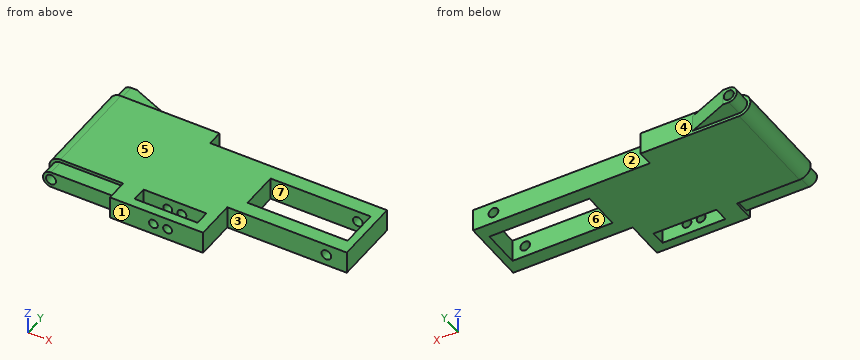
```python
from build123d import *

# Parameters (mm, degrees)
SKETCH_W        = 91.1
SKETCH_H        = 44.5
PAD_DEPTH       = 3.55
POCKET_DEPTH    = 7.101
SKETCH002_W     = 38
SKETCH002_H     = 12.8
POCKET001_DEPTH = 7.101
SKETCH003_W     = 23.5
SKETCH003_H     = 2
POCKET002_DEPTH = 7.101
SKETCH004_W     = 31.8
SKETCH004_H     = 12.2
POCKET003_DEPTH = 7.101
SKETCH005_W     = 20
SKETCH005_H     = 4.7
POCKET004_DEPTH = 7.101
POCKET005_DEPTH = 42.501
POCKET006_DEPTH = 5
POCKET007_DEPTH = 5.5
SKETCH009_R     = 1.6
POCKET008_DEPTH = 42.501
SKETCH010_R     = 1.55
POCKET009_DEPTH = 44.501
SKETCH011_R     = 1.4
POCKET010_DEPTH = 16


with BuildPart() as part:
    # Sketch → Pad (new body, symmetric)
    with BuildSketch(Plane.XY):
        with Locations((45.55, 0)):
            Rectangle(SKETCH_W, SKETCH_H)
    extrude(amount=PAD_DEPTH, both=True)

    # Sketch001 → Pocket (cut, through all)
    with BuildSketch(Plane.XY.offset(3.55)):
        Polygon((5.4, 22.25), (91.1, 22.25), (91.1, 11.85), (34.9, 11.85), (34.9, 16.75), (18.4, 16.75), align=None)
    extrude(amount=-POCKET_DEPTH, mode=Mode.SUBTRACT)

    # Sketch002 → Pocket001 (cut, through all)
    with BuildSketch(Plane.XY.offset(3.55)):
        with Locations((72.1, -15.85)):
            Rectangle(SKETCH002_W, SKETCH002_H)
    extrude(amount=-POCKET001_DEPTH, mode=Mode.SUBTRACT)

    # Sketch003 → Pocket002 (cut, through all)
    with BuildSketch(Plane.XY.offset(3.55)):
        with Locations((11.75, -21.25)):
            Rectangle(SKETCH003_W, SKETCH003_H)
    extrude(amount=-POCKET002_DEPTH, mode=Mode.SUBTRACT)

    # Sketch004 → Pocket003 (cut, through all)
    with BuildSketch(Plane.XY.offset(3.55)):
        with Locations((72.75, 1.15)):
            Rectangle(SKETCH004_W, SKETCH004_H)
    extrude(amount=-POCKET003_DEPTH, mode=Mode.SUBTRACT)

    # Sketch005 → Pocket004 (cut, through all)
    with BuildSketch(Plane.XY.offset(3.55)):
        with Locations((39.6, -17)):
            Rectangle(SKETCH005_W, SKETCH005_H)
    extrude(amount=-POCKET004_DEPTH, mode=Mode.SUBTRACT)

    # Sketch006 → Pocket005 (cut, through all)
    with BuildSketch(Plane.XZ.offset(20.25)):
        with BuildLine():
            Line((3.55, 3.55), (-1.45, 3.55))
            Line((-1.45, 3.55), (-1.45, -3.55))
            Line((-1.45, -3.55), (3.55, -3.55))
            ThreePointArc((3.55, 3.55), (0, 0), (3.55, -3.55))
        make_face()
    extrude(amount=-POCKET005_DEPTH, mode=Mode.SUBTRACT)

    # Sketch007 → Pocket006 (cut)
    with BuildSketch(Plane.XZ.offset(20.25)):
        with BuildLine():
            Line((0, 3.55), (23.5, 3.55))
            Line((23.5, 3.55), (23.5, 2.55))
            Line((23.5, 2.55), (3.55, 2.55))
            ThreePointArc((3.55, 2.55), (1, 0), (3.55, -2.55))
            Line((3.55, -2.55), (23.5, -2.55))
            Line((23.5, -2.55), (23.5, -3.55))
            Line((23.5, -3.55), (0, -3.55))
            Line((0, -3.55), (0, 3.55))
        make_face()
    extrude(amount=-POCKET006_DEPTH, mode=Mode.SUBTRACT)

    # Sketch008 → Pocket007 (cut)
    with BuildSketch(Plane(origin=(0, 22.25, 0), x_dir=(-1, 0, 0), z_dir=(0, 1, 0))):
        with BuildLine():
            Line((-18.4, 3.55), (0, 3.55))
            Line((0, 3.55), (0, -3.55))
            Line((0, -3.55), (-18.4, -3.55))
            Line((-18.4, -2.55), (-18.4, -3.55))
            Line((-3.55, -2.55), (-18.4, -2.55))
            ThreePointArc((-3.55, -2.55), (-1, 0), (-3.55, 2.55))
            Line((-18.4, 2.55), (-3.55, 2.55))
            Line((-18.4, 3.55), (-18.4, 2.55))
        make_face()
    extrude(amount=-POCKET007_DEPTH, mode=Mode.SUBTRACT)

    # Sketch009 → Pocket008 (cut, through all)
    with BuildSketch(Plane.XZ.offset(20.25)):
        with Locations((3.55, 0)):
            Circle(SKETCH009_R)
    extrude(amount=-POCKET008_DEPTH, mode=Mode.SUBTRACT)

    # Sketch010 → Pocket009 (cut, through all)
    with BuildSketch(Plane.XZ.offset(22.25)):
        with Locations((84.6, 0)):
            Circle(SKETCH010_R)
    extrude(amount=-POCKET009_DEPTH, mode=Mode.SUBTRACT)

    # Sketch011 → Pocket010 (cut)
    with BuildSketch(Plane.XZ.offset(22.25)):
        with Locations((41.8, 0)):
            Circle(SKETCH011_R)
        with Locations((37.3, 0)):
            Circle(SKETCH011_R)
    extrude(amount=-POCKET010_DEPTH, mode=Mode.SUBTRACT)


solid = part.part
```
Input: part model. Units: mm. Frame: model coordinates. Face numbers are marked on the shaded views. A direction names the side the tool comes from. Give positions to 0.01 mm unless a question says otherwise; leave off trailing zeros. Order: outer loops, then holes, each group sorted by start corner. A loop starts at its lowest first (then second) coordinate and runs counter-clockwise, first axis right, second up.
1. Set-up query: the marked faces 1, 2 and 3. Return all of +Z, -Z, +X, -X, +Y, -Y with unobstructed straight access to the full face (end or side cutting, diameter ignored); none if empty.
Computed:
face 1: +Z, -Z, +X, -X, -Y
face 2: +Z, -Z, +X, +Y
face 3: +Z, -Z, +X, -Y
2. Cut plane A-A (x = 37.3). Return loops of the section in (y, z), and give its area (3 significant figures).
Computed:
outline: (-22.25, -3.55) - (-19.35, -3.55) - (-19.35, -1.4) - (-22.25, -1.4) - close; (-22.25, 1.4) - (-19.35, 1.4) - (-19.35, 3.55) - (-22.25, 3.55) - close; (-14.65, -3.55) - (11.85, -3.55) - (11.85, 3.55) - (-14.65, 3.55) - (-14.65, 1.4) - (-6.25, 1.4) - (-6.25, -1.4) - (-14.65, -1.4) - close
area: 177 mm2
3. Draft query along Y for the marked faces 4, 5, 6 and 7. Return one class per face: released by +Y, released by -Y, zero draft, split by the parting line, or undercut.
Computed:
face 4: released by +Y
face 5: zero draft
face 6: undercut
face 7: undercut
4. Cut plane C-C (x = 63). Return loops of the section in (y, z).
Computed:
outline: (-9.45, -3.55) - (-4.95, -3.55) - (-4.95, 3.55) - (-9.45, 3.55) - close; (7.25, -3.55) - (11.85, -3.55) - (11.85, 3.55) - (7.25, 3.55) - close
5. Cut plane D-D (y = 8.5). Return loops of the section in (x, z), and give its area (3 significant figures).
Computed:
outline: (3.55, -3.55) - (91.1, -3.55) - (91.1, 3.55) - (3.55, 3.55) arc R3.55 ccw to start; hole circle Ø3.2 at (3.55, 0); hole circle Ø3.1 at (84.6, 0)
area: 626 mm2
6. Pin query (flat end, axial travel): pin 1 Ø1.5 at (x, y) = (18.5, -17.5) entering from -Z; pin 2 Ø1.5 at (y, z) = (15, -1.5) entering from +X; pin 3 Ø3.5 at (x, z) = (58.5, -1) entering from +Y; pin 4 Ø2.5 at (x, z) = (84.6, 0) entering from -Y (3 decimals). Return the tip coordinate at first contact, or that it passes through.
Computed:
pin 1: stops at z = -2.55
pin 2: stops at x = 34.9
pin 3: stops at y = 11.85
pin 4: passes through
7. Line query: probe 1 along Y at (x, z) = (61.5, -3); probe 2 along Z at (x, y) = (84.6, 10.6). Output: solid intervals per line, ascending.
Computed:
probe 1: y = -9.45 to -4.95, 7.25 to 11.85
probe 2: z = -3.55 to -1.55, 1.55 to 3.55
8. Cut plane B-B (y = 2.5). Return loops of the section in (x, z), and give its area (3 significant figures).
Computed:
outline: (3.55, -3.55) - (56.85, -3.55) - (56.85, 3.55) - (3.55, 3.55) arc R3.55 ccw to start; (88.65, -3.55) - (91.1, -3.55) - (91.1, 3.55) - (88.65, 3.55) - close; hole circle Ø3.2 at (3.55, 0)
area: 408 mm2
